Study the drawing (mm; zero at the part's minimum x, y, z) and answer. Coordinates: 2 decimals unless noted, no trailing zeros. Order: outer loops, then holes, each group sorted by start corner. A loop starts at its lowest first (then second) coordinate and runs counter-clockwise, first axis right, second up.
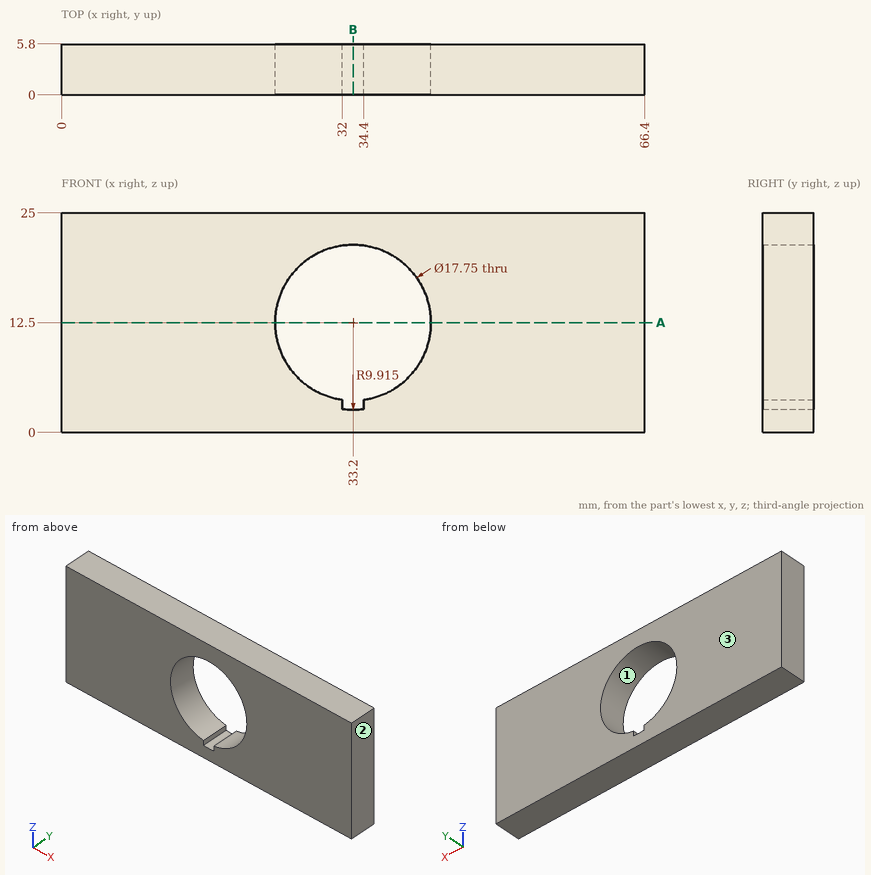
1) A cutting plane is placed at B-B, the plane x = 33.2. Determine the outline of the cut face in (y, z) (3 decimals).
A:
outline: (0, 0) - (5.8, 0) - (5.8, 2.585) - (0, 2.585) - close; (0, 21.375) - (5.8, 21.375) - (5.8, 25) - (0, 25) - close
2) Flat-ended cylindrical pins translate along their axes: pin 1 Ø6 at (x, z) = (39, 12.5) entering from +Y; pin 2 Ø1.5 at (y, z) = (4.5, 21.5) entering from -X. Find the tip coordinate at first contact, or state that the pin passes through.
A:
pin 1: passes through
pin 2: stops at x = 0
3) A cutting plane is placed at A-A, the plane z = 12.5. Determine the outline of the cut face in (x, y) (3 decimals), and give its area (3 significant figures).
A:
outline: (0, 0) - (24.325, 0) - (24.325, 5.8) - (0, 5.8) - close; (42.075, 0) - (66.4, 0) - (66.4, 5.8) - (42.075, 5.8) - close
area: 282 mm2
4) Determine the mould class of the marked faces 1, 2 and 3 for opening direction X: pulls with the +X half, pulls with the -X half, needs draft (parallel to the pull), parting line crosses it, or undercut.
A:
face 1: undercut
face 2: pulls with the +X half
face 3: needs draft
5) Straight lines are drawn through the part: line 1 (Z direction, x = 33.2, y = 4.35) (3 decimals); line 2 (X direction, y = 1.45, z = 12.5) (3 decimals); line 3 (X direction, y = 2.35, z = 7). For each, find the intervals that lie inside material, in ascending order.
A:
line 1: z = 0 to 2.585, 21.375 to 25
line 2: x = 0 to 24.325, 42.075 to 66.4
line 3: x = 0 to 26.23, 40.17 to 66.4
